```python
from build123d import *

# Parameters (mm, degrees)
SKETCH1_R           = 3.175
BOSS_EXTRUDE1_DEPTH = 9.525
CUT_EXTRUDE1_START  = -6.35
CUT_EXTRUDE1_DEPTH  = 6.35
FILLET1_R           = 6.35


with BuildPart() as part:
    # Sketch1 → Boss-Extrude1 (new, symmetric)
    with BuildSketch(Plane.XY):
        with BuildLine():
            Line((6.300964517, -0.787620565), (4.725723388, -13.389549599))
            Line((4.725723388, -13.389549599), (49.224758871, -18.951929034))
            Line((49.224758871, -18.951929034), (48.437138306, -25.252893551))
            Line((48.437138306, -25.252893551), (-2.362861694, -18.902893551))
            Line((-2.362861694, -18.902893551), (-0.787620565, -6.300964517))
            ThreePointArc((-0.787620565, -6.300964517), (-3.898522896, 5.01238658), (6.300964517, -0.787620565))
        make_face()
        with Locations(Location((0, 0, 0), (0, 0, 180))):
            Circle(SKETCH1_R, mode=Mode.SUBTRACT)
    extrude(amount=BOSS_EXTRUDE1_DEPTH, both=True)

    # Sketch2 → Cut-Extrude1 (cut)
    with BuildSketch(Plane.XY.offset(9.525).offset(CUT_EXTRUDE1_START)):
        Polygon((49.224758871, -18.951929034), (-15.764537124, -10.828267035), (-12.959816333, 11.60949929), (52.029479661, 3.485837291), align=None)
    extrude(amount=-CUT_EXTRUDE1_DEPTH, mode=Mode.SUBTRACT)

    # Fillet1
    fillet1_edges = [part.edges().sort_by_distance(p)[0] for p in [
        (-2.362861694, -18.902893551, 0),
    ]]
    fillet(fillet1_edges, radius=FILLET1_R - 0.0001)  # a hair under: the kernel refuses the full size


solid = part.part
```
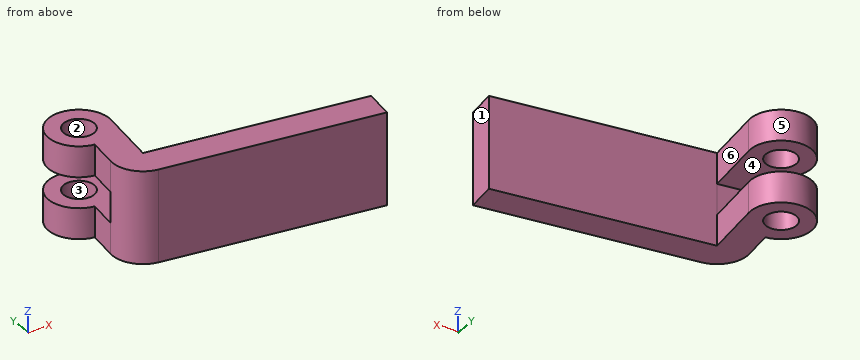
Source: CAD feature listing. Evaluate the final solid. Frame: model axes, mm. Face numbers are marked on the shaded views. A direction names the side the tool comes from. Round coordinates to 2 decimals unless told otherwise and drop trailing zeros. Loops run counter-clockwise (first coordinate to the right, second up) from the corner with the lowest first, then second, coordinate; pieces in that order, holes last. Notation, with made-up numbers: M 47,62 L 81,62 A25 ccw 81,94 Z; hole C 42,-18 d1. An arc over 180 degrees is marked long. Use a Markdown table: item, result. Add a question column.
1. Reachability of the marked faces 5 and 6 from +Z, -Z, +X, -X, +Y, -Y: full face, straight path, thin tool, end or side. Return the list, or none.
2. Section query C-C on y = -12. Return the cut outline in (x, z) (3 decimals).
3. Section query A-A on y = 0. Return the cut outline in (x, z) (3 decimals).
4. Section query D-D on x = 0. Return the cut outline in (y, z) (3 decimals).
5. Contact query for flat-ended pins moving along their axis: P1, Ø10, axis at x = 23, z = 3, coming from the -Y side; P2, Ø2, axis at y = -3.5, z = -7.5, coming from the -X side; P3, Ø1, axis at x = 29, z = -4, coming from the +Y side. Output: stop coordinate, or through.
6. Line query: line 1 (Z direction, x = -1.5, y = -12.5) (3 decimals); line 2 (Y direction, x = 0, z = 7) (3 decimals); line 3 (Y direction, x = 16, z = 3.25). Output: solid intervals per line, ascending.
7. Mould query, pull axis Y, two halves, no side actions, for the marked faces 1, 2, 3 and 4. Classes: pulls with the +Y half, pulls with the -Y half, needs draft (parallel to the pull), parting line crosses it, or undercut.
Reported:
| question | item | result |
|---|---|---|
| 1 | face 5 | +Z, -Z |
| 1 | face 6 | +Z, -Z, +X |
| 2 | outline | M -1.5,-9.525 L 4.899,-9.525 L 4.899,-3.175 L -1.5,-3.175 Z; M -1.5,3.175 L 4.899,3.175 L 4.899,9.525 L -1.5,9.525 Z |
| 3 | outline | M -6.35,-9.525 L -3.175,-9.525 L -3.175,-3.175 L -6.35,-3.175 Z; M -6.35,3.175 L -3.175,3.175 L -3.175,9.525 L -6.35,9.525 Z; M 3.175,-9.525 L 6.35,-9.525 L 6.35,-3.175 L 3.175,-3.175 Z; M 3.175,3.175 L 6.35,3.175 L 6.35,9.525 L 3.175,9.525 Z |
| 4 | outline | M -17.631,-9.525 L -3.175,-9.525 L -3.175,-3.175 L -12.799,-3.175 L -12.799,3.175 L -3.175,3.175 L -3.175,9.525 L -17.631,9.525 Z; M 3.175,-9.525 L 6.35,-9.525 L 6.35,-3.175 L 3.175,-3.175 Z; M 3.175,3.175 L 6.35,3.175 L 6.35,9.525 L 3.175,9.525 Z |
| 5 | P1 | stops at y = -22.7 |
| 5 | P2 | stops at x = -5.84 |
| 5 | P3 | stops at y = -16.36 |
| 6 | line 1 | z = -9.525 to -3.175, 3.175 to 9.525 |
| 6 | line 2 | y = -17.631 to -3.175, 3.175 to 6.35 |
| 6 | line 3 | y = -21.2 to -14.8 |
| 7 | face 1 | pulls with the -Y half |
| 7 | face 2 | undercut |
| 7 | face 3 | undercut |
| 7 | face 4 | needs draft |
